from build123d import *

# Parameters (mm, degrees)
MDFESB_W        = 200
MDFESB_H        = 75
MDF_DEPTH       = 3
ENTRADASESB_W   = 10
ENTRADASESB_H   = 3
ENTRADASESB_W_2 = 3
ENTRADASESB_H_2 = 10
ENTRADAS_DEPTH  = 3


with BuildPart() as part:
    # mdfEsb → mdf (new body)
    with BuildSketch(Plane(origin=(0, 0, 0), x_dir=(0, 0, -1), z_dir=(1, 0, 0))):
        with Locations((100, 37.5)):
            Rectangle(MDFESB_W, MDFESB_H)
    extrude(amount=MDF_DEPTH)

    # entradasEsb → Entradas (cut)
    with BuildSketch(Plane(origin=(3, 0, 0), x_dir=(0, 0, -1), z_dir=(1, 0, 0))):
        with Locations((15, 1.5)):
            Rectangle(ENTRADASESB_W, ENTRADASESB_H)
        with Locations((35, 1.5)):
            Rectangle(ENTRADASESB_W, ENTRADASESB_H)
        with Locations((55, 1.5)):
            Rectangle(ENTRADASESB_W, ENTRADASESB_H)
        with Locations((75, 1.5)):
            Rectangle(ENTRADASESB_W, ENTRADASESB_H)
        with Locations((95, 1.5)):
            Rectangle(ENTRADASESB_W, ENTRADASESB_H)
        with Locations((115, 1.5)):
            Rectangle(ENTRADASESB_W, ENTRADASESB_H)
        with Locations((135, 1.5)):
            Rectangle(ENTRADASESB_W, ENTRADASESB_H)
        with Locations((155, 1.5)):
            Rectangle(ENTRADASESB_W, ENTRADASESB_H)
        with Locations((175, 1.5)):
            Rectangle(ENTRADASESB_W, ENTRADASESB_H)
        with Locations((198.5, 25)):
            Rectangle(ENTRADASESB_W_2, ENTRADASESB_H_2)
        with Locations((198.5, 45)):
            Rectangle(ENTRADASESB_W_2, ENTRADASESB_H_2)
        with Locations((198.5, 65)):
            Rectangle(ENTRADASESB_W_2, ENTRADASESB_H_2)
        Polygon((190, 0), (190, 3), (197, 3), (197, 10), (200, 10), (200, 0), align=None)
        with Locations((185, 73.5)):
            Rectangle(ENTRADASESB_W, ENTRADASESB_H)
        with Locations((165, 73.5)):
            Rectangle(ENTRADASESB_W, ENTRADASESB_H)
    extrude(amount=-ENTRADAS_DEPTH, mode=Mode.SUBTRACT)


solid = part.part
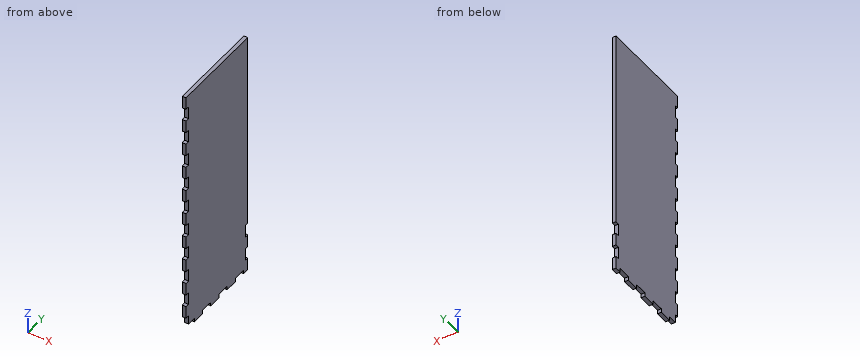
Geometry: final body of the model. Coordinates: model frame, mm. Give positions to 0.01 mm unless a question says otherwise; leave off trailing zeros. Write each loop counter-clockwise with the first axis right and the second up, starting at its lowest first coordinate (ties: lowest second). Pieces come first, ordered by that corner, then holes. Notation, with made-up numbers: (0.25, 68.5) - (49.25, 68.5) arc R18 ccw to (49.25, 82.5) - close; hole circle Ø6 at (41, 83). An arc over 180 degrees is marked (long way). Return JSON: item names as keys, results as strings. Group by question number.
1) Section B-B on z = -96. Return the cut outline in (x, y), plus the area to 3 significant figures.
2) Section A-A on y = 47. Return the cut outline in (x, z), plus the area to 3 significant figures.
3) Line query: line 1 (Y direction, x = 2.3, z = -183.5); line 2 (Y direction, x = 2.5, z = -34.5); line 3 (Z direction, x = 2.2, y = 41.5). Output: solid intervals per line, ascending.
4) First-contact query: P1, Ø0.9, axis at x = 1.5, y = 26.5, coming from the -Z side; P2, Ø1.5, axis at x = 1.5, y = 1.5, coming from the +Z side; P3, Ø0.9, axis at x = 2, y = 1, coming from the -Z side. Flat tips, straight axial feed; report the tip coordinate or a pass-through.
Filled in:
{
 "1": {"outline": "(0, 3) - (3, 3) - (3, 75) - (0, 75) - close", "area": "216 mm^2"},
 "2": {"outline": "(0, -197) - (3, -197) - (3, 0) - (0, 0) - close", "area": "591 mm^2"},
 "3": {"line 1": "y = 0 to 72", "line 2": "y = 3 to 75", "line 3": "z = -197 to 0"},
 "4": {"P1": "stops at z = -197", "P2": "stops at z = 0", "P3": "stops at z = -190"}
}
